from build123d import *

# Parameters (mm, degrees)
BOSS_EXTRUDE1_DEPTH      = 40
SKETCH3_W                = 125
SKETCH3_H                = 40
BOSS_EXTRUDE2_DEPTH      = 5
BOSS_EXTRUDE2_DEPTH_BACK = 5
SKETCH4_W                = 10
SKETCH4_H                = 10
BOSS_EXTRUDE3_DEPTH      = 20
BOSS_EXTRUDE3_TAPER      = 7


with BuildPart() as part:
    # Sketch2 → Boss-Extrude1 (new body)
    with BuildSketch(Plane(origin=(0, 0, 0), x_dir=(1, 0, 0), z_dir=(0, 1, 0))):
        Polygon((-10, 7.5), (-10, -7.5), (-5, -7.5), (-5, -2.5), (0, -2.5), (0, 2.5), (-5, 2.5), (-5, 7.5), align=None)
    extrude(amount=BOSS_EXTRUDE1_DEPTH)

    # Sketch3 → Boss-Extrude2 (add, two sides)
    with BuildSketch(Plane.XY) as boss_extrude2_sk:
        with Locations((62.5, 20)):
            Rectangle(SKETCH3_W, SKETCH3_H)
    extrude(amount=BOSS_EXTRUDE2_DEPTH)
    extrude(boss_extrude2_sk.sketch, amount=-BOSS_EXTRUDE2_DEPTH_BACK)

    # Sketch4 → Boss-Extrude3 (add)
    with BuildSketch(Plane.XZ):
        with Locations((120, 0)):
            Rectangle(SKETCH4_W, SKETCH4_H)
    extrude(amount=BOSS_EXTRUDE3_DEPTH, taper=BOSS_EXTRUDE3_TAPER)


solid = part.part
Design review of the part built by this model. Coordinates are the model's own, in mm. A direction names the side the tool comes from. Give positions to 0.01 mm unless a question says otherwise; leave off trailing zeros. Write each loop counter-clockwise with the first axis right and the second up, starting at its lowest first coordinate (ties: lowest second). Pieces come first, ordered by that corner, then holes. Notation, with made-up numbers: M 24.5,72.5 L 68.5,72.5 A18 ccw 68.5,104.5 Z; hole C 27.25,29 d10. An arc over 180 degrees is marked long. Answer as a JSON object with one key per item and string values. Group by question number.
1) Mouldability with a two-part tool opening along X and no side actions: class faces 1 (the face through (-5, 20, 5)), 2 (the face through (120, -20, 0)), 3 (the face through (125, 20, 0)), 4 (the face through (-5, 20, -5)) as released by +X, released by -X, zero draft, split by the parting line, or undercut.
2) We need section A-A (y = 9). Give the boundary of the cut face in (x, z), and give its area (3 significant figures).
3) Tool access review of faces 5 (the face through (62, 20, 5)), 6 (the face through (52, 0, 0)), 7 (the face through (62, 20, -5)), 8 (the face through (0, 20, -4)), 9 (the face through (-3, 20, 2.5)): name each direction out of +Z, -Z, +X, -X, +Y, -Y from which nothing blocks a thin tool from reaching the whole face with its end or side.
4) We need section B-B (x = 40). Give the boundary of the cut face in (y, z).
5) Clearance check with flat-ended pins moving along their axes: pin 1 Ø3 at (y, z) = (-3.5, -2.5) entering from +X; pin 2 Ø12 at (x, y) = (35, 30) entering from +Z; pin 3 Ø4 at (x, z) = (100.5, -1.5) entering from -Y. State where each tip first meets the part, or that it passes through.
6) For line 1 along X through (y, z) = (23, 4.25); line 2 along Z through (x, y) = (40, 1.5); line 3 along Y through (x, z) = (70.5, 1), list the stretches that pass through material, from the lowest coordinate up.
Answer key:
{
 "1": {"face 1": "undercut", "face 2": "zero draft", "face 3": "released by +X", "face 4": "undercut"},
 "2": {"outline": "M -10,-7.5 L -5,-7.5 L -5,-2.5 L 0,-2.5 L 0,-5 L 125,-5 L 125,5 L 0,5 L 0,2.5 L -5,2.5 L -5,7.5 L -10,7.5 Z", "area": "1,350 mm²"},
 "3": {"face 5": "+Z, +X, +Y, -Y", "face 6": "+Z, -Z, -X, -Y", "face 7": "-Z, +X, +Y, -Y", "face 8": "-Z, +Y, -Y", "face 9": "+Z, +Y, -Y"},
 "4": {"outline": "M 0,-5 L 40,-5 L 40,5 L 0,5 Z"},
 "5": {"pin 1": "stops at x = 124.75", "pin 2": "stops at z = 5", "pin 3": "stops at y = 0"},
 "6": {"line 1": "x = -10 to -5, 0 to 125", "line 2": "z = -5 to 5", "line 3": "y = 0 to 40"}
}
